```python
from build123d import *

# Parameters (mm, degrees)
F1_DEPTH = 6.35


with BuildPart() as f1:
    # F0 (on Top) → F1 (new body)
    with BuildSketch(Plane.XY):
        with BuildLine():
            Line((-1.125735, 22.943184), (-20.32, -10.302259))
            Line((-20.32, -10.302259), (0, -10.302259))
            Line((0, -10.302259), (20.32, -10.302259))
            Line((20.32, -10.302259), (1.125735, 22.943184))
            ThreePointArc((1.125735, 22.943184), (0, 27.144483), (-1.125735, 22.943184))
        make_face()
        with BuildLine():
            Line((-0.764991, -9.103689), (-18.208449, -9.103689))
            Line((-18.208449, -9.103689), (-9.496779, 5.985365))
            ThreePointArc((-9.496779, 5.985365), (-9.171397, -3.89734), (-0.764991, -9.103689))
        make_face(mode=Mode.SUBTRACT)
        with BuildLine():
            Line((-0.764991, 10.540828), (-0.764991, -7.850349))
            ThreePointArc((-0.764991, -7.850349), (-9.174241, 1.345239), (-0.764991, 10.540828))
        make_face(mode=Mode.SUBTRACT)
        with BuildLine():
            ThreePointArc((0.764991, -9.103689), (9.171397, -3.89734), (9.496779, 5.985365))
            Line((9.496779, 5.985365), (18.208449, -9.103689))
            Line((18.208449, -9.103689), (0.764991, -9.103689))
        make_face(mode=Mode.SUBTRACT)
        with BuildLine():
            Line((0.764991, -7.850349), (0.764991, 10.540828))
            ThreePointArc((0.764991, 10.540828), (9.174241, 1.345239), (0.764991, -7.850349))
        make_face(mode=Mode.SUBTRACT)
        with BuildLine():
            Line((-0.764991, 21.109266), (-0.764991, 11.799275))
            ThreePointArc((-0.764991, 11.799275), (-5.334498, 10.422163), (-8.818391, 7.160368))
            Line((-8.818391, 7.160368), (-0.764991, 21.109266))
        make_face(mode=Mode.SUBTRACT)
        with BuildLine():
            ThreePointArc((8.818391, 7.160368), (5.334498, 10.422163), (0.764991, 11.799275))
            Line((0.764991, 11.799275), (0.764991, 21.109266))
            Line((0.764991, 21.109266), (8.818391, 7.160368))
        make_face(mode=Mode.SUBTRACT)
        with BuildLine():
            ThreePointArc((1.583799, 24.893014), (1.37161, 24.101114), (0.7919, 23.521403))
            ThreePointArc((0.7919, 23.521403), (0, 23.309214), (-0.7919, 23.521403))
            ThreePointArc((-0.7919, 23.521403), (-0.7919, 26.264624), (1.583799, 24.893014))
        make_face(mode=Mode.SUBTRACT)
    extrude(amount=F1_DEPTH)


solid = f1.part
```
Can you work these out from the model? Positions are in its coordinate system, mm. A direction names the side the tool comes from. Coordinates: 2 decimals unless noted, no trailing zeros. Loops run counter-clockwise (first coordinate to the right, second up) from the corner with the lowest first, then second, coordinate; pieces in that order, holes last. Notation, with made-up numbers: M 58,54 L 69,54 A14 ccw 69,71 Z; hole C 56.5,48 d2. An arc over 180 degrees is marked long. Put each result on its own line as item: value. Start each with the question number.
(1) Will these pins go through, and if not, where does the flat tip stop? pin 1 Ø1.5 at (x, z) = (-8.5, 4.5) entering from +Y; pin 2 Ø1.9 at (y, z) = (2.5, 3) entering from +X; pin 3 Ø1.9 at (y, z) = (5, 4.5) entering from -X.
(2) Imagine slicing it at C-C on y = 2. List the corners of the cut face in (x, z) for me (3 decimals).
(3) Imagine slicing it at D-D on x = 12.5. List the corners of the cut face in (y, z) for me, and give its area (3 significant figures).
(4) We'd pull the mould along X, two halves only. Please class faces 3 (the face through (-0.765, 17, 3)), 4 (the face through (10.857, 6.088, 3.131)), 5 (the face through (0, 3, 6.35)), 6 (the face through (-9.172, 1.154, 3.131)): +X half, -X half, draft (parallel to the pull), parting line (faces both ways), or undercut.
(5) Imagine slicing it at B-B on x = 0. List the corners of the cut face in (y, z) for me, and give its area (3 significant figures).
(6) I need wall thicknesses on probe 1 along Y at (x, z) = (0, 3); probe 2 along X at (y, z) = (0.5, 2) (3 decimals); probe 3 along X at (y, z) = (8.5, 1.25) (3 decimals). Which ranges of each line are inside material? Lowest first, please.
(7) Imagine slicing it at A-A on z = 3.75. List the corners of the cut face in (x, y) for me (1 decimal).
(8) Which directions (+Z, -Z, +X, -X, +Y, -Y) give clear straight access to the entire face, cutting with the end or side of a thin tool? Please do faces 1 (the face through (0.765, 1, 3)), 2 (the face through (0, 3, 0)).
Worked answers:
1. pin 1: stops at y = 11.47
1. pin 2: stops at x = 13.48
1. pin 3: stops at x = -12.03
2. outline: M -13.217,0 L -11.798,0 L -11.798,6.35 L -13.217,6.35 Z; M -10.559,0 L -9.151,0 L -9.151,6.35 L -10.559,6.35 Z; M -0.765,0 L 0.765,0 L 0.765,6.35 L -0.765,6.35 Z; M 9.151,0 L 10.559,0 L 10.559,6.35 L 9.151,6.35 Z; M 11.798,0 L 13.217,0 L 13.217,6.35 L 11.798,6.35 Z
3. outline: M -10.3,0 L -9.1,0 L -9.1,6.35 L -10.3,6.35 Z; M 0.78,0 L 3.24,0 L 3.24,6.35 L 0.78,6.35 Z
3. area: 23.2 mm2
4. face 3: undercut
4. face 4: +X half
4. face 5: draft
4. face 6: undercut
5. outline: M -10.3,0 L 23.31,0 L 23.31,6.35 L -10.3,6.35 Z; M 26.48,0 L 27.14,0 L 27.14,6.35 L 26.48,6.35 Z
5. area: 218 mm2
6. probe 1: y = -10.3 to 23.31, 26.48 to 27.14
6. probe 2: x = -14.083 to -12.664, -10.545 to -9.135, -0.765 to 0.765, 9.135 to 10.545, 12.664 to 14.083
6. probe 3: x = -9.465 to -8.045, -7.757 to -5.777, -0.765 to 0.765, 5.777 to 7.757, 8.045 to 9.465
7. outline: M -20.3,-10.3 L 20.3,-10.3 L 1.1,22.9 A2.3 ccw long -1.1,22.9 Z; hole M -18.2,-9.1 L -0.8,-9.1 A10.5 cw -9.5,6 Z; hole M -8.8,7.2 A10.5 cw -0.8,11.8 L -0.8,21.1 Z; hole M -0.8,-7.9 L -0.8,10.5 A9.2 ccw Z; hole M 0.8,-9.1 L 18.2,-9.1 L 9.5,6 A10.5 cw Z; hole M 0.8,-7.9 A9.2 ccw 0.8,10.5 Z; hole M 0.8,11.8 A10.5 cw 8.8,7.2 L 0.8,21.1 Z; hole M 0.8,23.5 A1.6 ccw 1.6,24.9 A1.6 ccw long Z
8. face 1: +Z, -Z
8. face 2: -Z, +X, -X, +Y, -Y
